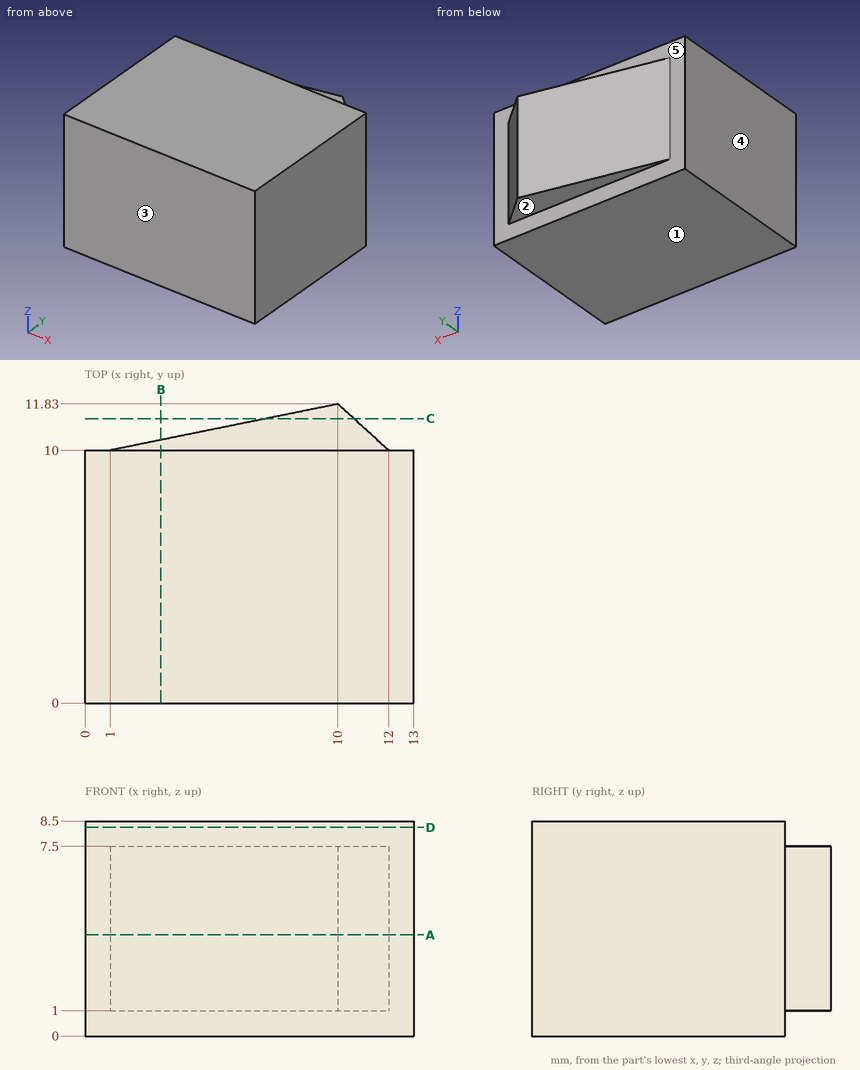
Answer from the drawing. Dimensions are ordinates in mm from the lowest x, y and z of the part. A direction names the side the tool comes from. Coordinates: 2 decimals unless noted, no trailing zeros. Loops run counter-clockwise (first coordinate to the right, second up) from the corner with the lowest first, then second, coordinate; pieces in that order, holes last. Notation, with made-up numbers: (-37.75, -28.75) -> (-19.75, -28.75) arc R17 cw to (-19.75, -11.75) -> close; hole circle Ø6 at (4, 48.25). An arc over 180 degrees is marked (long way). Answer in a Markdown table with one row per item.
Item 1: A cutting plane is placed at A-A on z = 4. Determine the outline of the cut face in (x, y).
Returned:
| item | result |
|---|---|
| outline | (0, 0) -> (13, 0) -> (13, 10) -> (12, 10) -> (10, 11.83) -> (1, 10) -> (0, 10) -> close |
Item 2: A cutting plane is placed at C-C on y = 11.25. Determine the outline of the cut face in (x, z).
Returned:
| item | result |
|---|---|
| outline | (7.15, 1) -> (10.63, 1) -> (10.63, 7.5) -> (7.15, 7.5) -> close |
Item 3: This flat-tipped pin is pushed along its axis until it touches: P1, Ø1.5, axis at x = 7.5, y = 11, coming from the +Z side. Where does it stop, or does it pass through?
Returned:
| item | result |
|---|---|
| P1 | stops at z = 7.5 |
Item 4: A cutting plane is placed at B-B on x = 3. Determine the outline of the cut face in (y, z).
Returned:
| item | result |
|---|---|
| outline | (0, 0) -> (10, 0) -> (10, 1) -> (10.41, 1) -> (10.41, 7.5) -> (10, 7.5) -> (10, 8.5) -> (0, 8.5) -> close |
Item 5: For the marked faces 1 and 2, determine the directions among +Z, -Z, +X, -X, +Y, -Y from which every point of the face is accessible in a straight line to the end or side of a thin tool.
Returned:
| item | result |
|---|---|
| face 1 | -Z, +X, -X, +Y, -Y |
| face 2 | -Z, +X, -X, +Y |
Item 6: A cutting plane is placed at D-D on z = 8.25. Determine the outline of the cut face in (x, y).
Returned:
| item | result |
|---|---|
| outline | (0, 0) -> (13, 0) -> (13, 10) -> (0, 10) -> close |
Item 7: For a pull along Y with two mould halves and no side action, classify the marked faces 3, 4 and 5 as released by +Y, released by -Y, zero draft, split by the parting line, or undercut.
Returned:
| item | result |
|---|---|
| face 3 | released by -Y |
| face 4 | zero draft |
| face 5 | released by +Y |
Item 8: Straight lines are drawn through the part: line 1 along Y through (x, z) = (1, 4.25); line 2 along Y through (x, z) = (10.25, 2.5). For each, find the intervals that lie inside material, in ascending order. Write a range as [from, to].
Returned:
| item | result |
|---|---|
| line 1 | y = [0, 10] |
| line 2 | y = [0, 11.6] |
